Here's how the part is built. I have some questions about the finished solid (model axes, mm). Face numbers are marked on the shaded views. A direction names the side the tool comes from. Give positions to 0.01 mm unless a question says otherwise; leave off trailing zeros. Order: outer loops, then holes, each group sorted by start corner. A loop starts at its lowest first (then second) coordinate and runs counter-clockwise, first axis right, second up. Notation, with made-up numbers: M 41.5,-40 L 82.5,-40 A33 cw 82.5,-3 Z; hole C -28,23.5 d3. An arc over 180 degrees is marked long. Use one line per item in the form item = value.
from build123d import *

# Parameters (mm, degrees)
F0_W     = 50
F0_H     = 50
F1_DEPTH = 52
F2_W     = 50
F2_H     = 1.5
F3_DEPTH = 42
F5_DEPTH = 36
F6_R     = 6.680851
F7_DEPTH = 65.6
F8_R     = 10
F9_DEPTH = 12


with BuildPart() as f1:
    # F0 (on Right) → F1 (new body)
    with BuildSketch(Plane.YZ):
        with Locations((-25, 25)):
            Rectangle(F0_W, F0_H)
    extrude(amount=F1_DEPTH)

    # F2 (on face) → F3 (cut)
    with BuildSketch(Plane.YZ.offset(52)):
        with Locations((-25, 0.75)):
            Rectangle(F2_W, F2_H)
    extrude(amount=-F3_DEPTH, mode=Mode.SUBTRACT)

    # F4 (on face) → F5 (cut)
    with BuildSketch(Plane(origin=(0, 0, 1.5), x_dir=(1, 0, 0), z_dir=(0, 0, -1))):
        with BuildLine():
            Line((68.967977, -80.566245), (77.262936, 141.644415))
            ThreePointArc((77.262936, 141.644415), (36.12911, 31.919758), (68.967977, -80.566245))
        make_face()
    extrude(amount=-F5_DEPTH, mode=Mode.SUBTRACT)

    # F6 (on face) → F7 (cut)
    with BuildSketch(Plane.XY.offset(50)):
        with Locations((22, -25)):
            Circle(F6_R)
    extrude(amount=-F7_DEPTH, mode=Mode.SUBTRACT)

    # F8 (on face) → F9 (cut)
    with BuildSketch(Plane.XY.offset(50)):
        with Locations((22, -25)):
            Circle(F8_R)
    extrude(amount=-F9_DEPTH, mode=Mode.SUBTRACT)


solid = f1.part
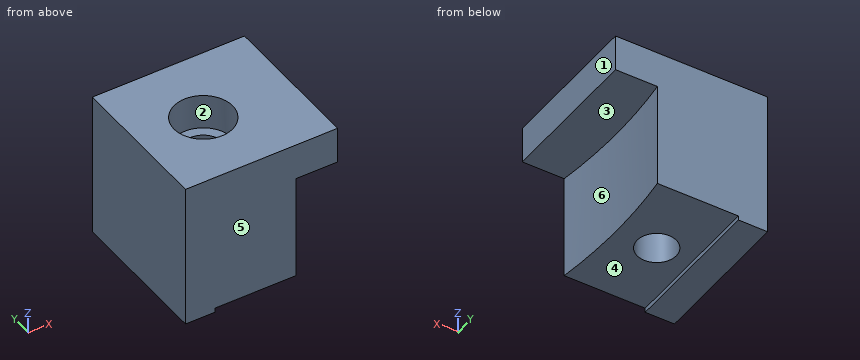
Q1. I want a section at B-B on y = -25. Write out the boundary of the cut face in (x, z), then the cut area to 3 significant figures.
Found:
outline = M 0,0 L 10,0 L 10,1.5 L 15.32,1.5 L 15.32,38 L 12,38 L 12,50 L 0,50 Z; M 28.68,1.5 L 36,1.5 L 36,37.5 L 52,37.5 L 52,50 L 32,50 L 32,38 L 28.68,38 Z
area = 1,230 mm²
Q2. Thinking about a two-plate mould opening in X: for the marked faces 1, 2 and 3, which applies, +X half, -X half, draft (parallel to the pull), parting line (faces both ways), or undercut?
Found:
face_1 = +X half
face_2 = undercut
face_3 = draft
Q3. On a 3-axis mill with a long thin cutter (end or side, diameter ignored), from which of +Z, -Z, +X, -X, +Y, -Y can I reach the whole of each face in a straight line? I mean the marked faces 4, 5 and 6. Say none if no direction works.
Found:
face_4 = -Z, +X, +Y, -Y
face_5 = +Z, -Z, +X, -X, -Y
face_6 = -Z, +X
Q4. I want a section at C-C on z = 29.5. Write out the boundary of the cut face in (x, y).
Found:
outline = M 0,-50 L 37.69,-50 A185.5 cw 37.69,0 L 0,0 Z; hole C 22,-25 d13.36
Q5. I need wall thicknesses on L1, parallel to Y at x = 22, z = 46.75; L2, parallel to Y at x = 22, z = 25; L3, parallel to Z at x = 40, y = -25. Which ranges of each line are inside material? Lowest first, please.
Found:
L1 = -50 to -35, -15 to 0
L2 = -50 to -31.68, -18.32 to 0
L3 = 37.5 to 50
Q6. I want a section at A-A on x = 22. Write out the boundary of the cut face in (y, z).
Found:
outline = M -50,1.5 L -31.68,1.5 L -31.68,38 L -35,38 L -35,50 L -50,50 Z; M -18.32,1.5 L 0,1.5 L 0,50 L -15,50 L -15,38 L -18.32,38 Z
Q7. I want a section at D-D on x = 30. Write out the boundary of the cut face in (y, z), then the cut area to 3 significant figures.
Found:
outline = M -50,1.5 L 0,1.5 L 0,50 L -19,50 L -19,38 L -31,38 L -31,50 L -50,50 Z
area = 2,280 mm²
Q8. I'm going to push flat-ended pins straight in: pin 1 Ø12 at (x, y) = (22, -25) entering from -Z; pin 2 Ø8 at (x, y) = (40, -17.5) entering from -Z; pin 3 Ø17.5 at (x, y) = (22, -25) entering from +Z; pin 4 Ø12 at (y, z) = (-8, 12) entering from +X. Where does each tip first touch, or does it pass through?
Found:
pin_1 = through
pin_2 = 1.5
pin_3 = 38
pin_4 = 37.43
